Work out the finished part from the listing and answer in its coordinate system (mm). A direction names the side the tool comes from. Round coordinates to 2 decimals unless told otherwise and drop trailing zeros. Order: outer loops, then holes, each group sorted by start corner. A loop starts at its lowest first (then second) coordinate and runs counter-clockwise, first axis right, second up. Notation, with made-up numbers: M -38.75,-15 L -17.75,-15 A33 ccw -17.75,16 Z; hole C 87,-32 d4. An arc over 180 degrees is marked long. Return JSON: item names as keys, results as strings.
from build123d import *

# Parameters (mm, degrees)
SKETCH1_W                   = 30
SKETCH1_H                   = 30
SKETCH1_W_2                 = 25
SKETCH1_H_2                 = 25
BOSS_EXTRUDE1_DEPTH         = 300
F_1_4_0_25_DIAMETER_HOLE1_D = 6.35
CUT_EXTRUDE1_DEPTH          = 302.869176962
CUT_EXTRUDE2_DEPTH          = 302.869176962


with BuildPart() as part:
    # Sketch1 → Boss-Extrude1 (new body)
    with BuildSketch(Plane(origin=(0, 0, 0), x_dir=(1, 0, 0), z_dir=(0, 1, 0))):
        Rectangle(SKETCH1_W, SKETCH1_H)
        Rectangle(SKETCH1_W_2, SKETCH1_H_2, mode=Mode.SUBTRACT)
    extrude(amount=BOSS_EXTRUDE1_DEPTH)

    # 1/4 (0.25) Diameter Hole1 (through all)
    with Locations(Plane.ZY.offset(15)):
        with Locations((0, 15)):
            Hole(F_1_4_0_25_DIAMETER_HOLE1_D / 2)

    # Sketch4 → Cut-Extrude1 (cut, through all)
    with BuildSketch(Plane.ZY.offset(15)):
        with BuildLine():
            Line((-10, 300), (-10, 290))
            ThreePointArc((-10, 290), (-0.626229125, 280.019627408), (9.921567416, 288.75))
            Line((9.921567416, 288.75), (15, 288.75))
            Line((15, 288.75), (15, 300))
            Line((15, 300), (-10, 300))
        make_face()
    extrude(amount=-CUT_EXTRUDE1_DEPTH, mode=Mode.SUBTRACT)

    # Sketch5 → Cut-Extrude2 (cut, through all)
    with BuildSketch(Plane.ZY.offset(15)):
        with BuildLine():
            Line((-3.122162674, 15.576823403), (-6, 0))
            Line((-6, 0), (6, 0))
            Line((6, 0), (3.122162674, 15.576823403))
            ThreePointArc((3.122162674, 15.576823403), (0, 18.175), (-3.122162674, 15.576823403))
        make_face()
    extrude(amount=-CUT_EXTRUDE2_DEPTH, mode=Mode.SUBTRACT)


solid = part.part
Item 1: Find section B-B (z = 0). Determine the outline of the cut face in (x, y) (3 decimals).
Output:
{"outline": "M -15,18.175 L -12.5,18.175 L -12.5,280 L -15,280 Z; M 12.5,18.175 L 15,18.175 L 15,280 L 12.5,280 Z"}
Item 2: Find section C-C (y = 219.5). Determine the outline of the cut face in (x, z).
Output:
{"outline": "M -15,-15 L 15,-15 L 15,15 L -15,15 Z; hole M -12.5,-12.5 L 12.5,-12.5 L 12.5,12.5 L -12.5,12.5 Z"}
Item 3: Find section A-A (x = -1). Determine the outline of the cut face in (y, z), plus the area to 3 significant figures.
Output:
{"outline": "M 0,-15 L 300,-15 L 300,-12.5 L 0,-12.5 Z; M 0,12.5 L 288.75,12.5 L 288.75,15 L 0,15 Z", "area": "1,470 mm^2"}
Item 4: Consider line 1 along X through (y, z) = (260, -7); line 2 along Y through (x, z) = (2.75, 13). Determine where each line is inside the solid, lowest interval first. Write a range as [from, to].
Output:
{"line 1": "x = [-15, -12.5], [12.5, 15]", "line 2": "y = [0, 288.75]"}
Item 5: Which of the six approach directions +Z, -Z, +X, -X, +Y, -Y give full straight-line access (tool end or side, diameter ignored) to faces 1 (the flat face through (0, 148, -12.5)), 2 (the flat face through (0, 0, -13)), 3 (the flat face through (0, 288.75, 14))?
Output:
{"face 1": "+Y, -Y", "face 2": "+Z, -Z, +X, -X, -Y", "face 3": "+Z, +X, -X, +Y"}
Item 6: Each of these flat-tipped pins is pushed along its axis until it touches: pin 1 (0.8 mm diameter, centred on x = 14.5, y = 296, fed in from +Z); pin 2 (4 mm diameter, centred on x = 0, z = 12, fed in from +Y); pin 3 (3 mm diameter, centred on x = 10, z = 3.5, fed in from -Y). Where does it stop, or does it pass through?
Output:
{"pin 1": "stops at z = -10", "pin 2": "stops at y = 288.75", "pin 3": "passes through"}
Item 7: The mould has two halves that part along Z. Classify faces 4 (the flat face through (0, 142, 15)), 5 (the cylindrical face through (13.733, 280.035, -0.837)), 6 (the flat face through (0, 0, 13)): pulls with the +Z half, pulls with the -Z half, needs draft (parallel to the pull), parting line crosses it, or undercut.
Output:
{"face 4": "pulls with the +Z half", "face 5": "undercut", "face 6": "needs draft"}
